Geometry: final body of the model. Coordinates: model frame, mm. A direction names the side the tool comes from. Give positions to 0.01 mm unless a question says otherwise; leave off trailing zeros. Loops run counter-clockwise (first coordinate to the right, second up) from the corner with the lowest first, then second, coordinate; pieces in that order, holes last.
from build123d import *

# Parameters (mm, degrees)
EXTRUDE_1_DEPTH = 4.5


with BuildPart() as part:
    # 草图1 → 凸台-拉伸1 (new body)
    with BuildSketch(Plane(origin=(0, 0, 0), x_dir=(1, 0, 0), z_dir=(0, 1, 0))):
        with BuildLine():
            Line((-6.23452468, 62.552230204), (0.89047532, 62.552230204))
            Line((0.89047532, 62.552230204), (0.89047532, 67.052230204))
            Line((0.89047532, 67.052230204), (8.01547532, 67.052230204))
            Line((8.01547532, 67.052230204), (8.01547532, 62.552230204))
            Line((8.01547532, 62.552230204), (15.14047532, 62.552230204))
            Line((15.14047532, 62.552230204), (15.14047532, 67.052230204))
            Line((15.14047532, 67.052230204), (22.26547532, 67.052230204))
            Line((22.26547532, 67.052230204), (22.26547532, 62.552230204))
            Line((22.26547532, 62.552230204), (29.39047532, 62.552230204))
            Line((29.39047532, 62.552230204), (29.39047532, 55.427230204))
            Line((29.39047532, 55.427230204), (33.89047532, 55.427230204))
            Line((33.89047532, 55.427230204), (33.89047532, 48.302230204))
            Line((33.89047532, 48.302230204), (29.39047532, 48.302230204))
            Line((29.39047532, 48.302230204), (29.39047532, 41.177230204))
            Line((29.39047532, 41.177230204), (33.89047532, 41.177230204))
            Line((33.89047532, 41.177230204), (33.89047532, 34.052230204))
            Line((33.89047532, 34.052230204), (29.39047532, 34.052230204))
            Line((29.39047532, 34.052230204), (29.39047532, 26.927230204))
            Line((29.39047532, 26.927230204), (33.89047532, 26.927230204))
            Line((33.89047532, 26.927230204), (33.89047532, 19.802230204))
            Line((33.89047532, 19.802230204), (29.39047532, 19.802230204))
            Line((29.39047532, 19.802230204), (29.39047532, 12.677230204))
            Line((29.39047532, 12.677230204), (33.89047532, 12.677230204))
            Line((33.89047532, 12.677230204), (33.89047532, 5.552230204))
            Line((33.89047532, 5.552230204), (29.39047532, 5.552230204))
            Line((29.39047532, 5.552230204), (29.39047532, -34.999800679))
            ThreePointArc((29.39047532, -34.999800679), (29.238234385, -35.765167544), (28.804688882, -36.414014242))
            Line((28.804688882, -36.414014242), (28.476261758, -36.742441366))
            ThreePointArc((28.476261758, -36.742441366), (28.042716255, -37.391288064), (27.89047532, -38.156654929))
            Line((27.89047532, -38.156654929), (27.89047532, -49.877331374))
            ThreePointArc((27.89047532, -49.877331374), (27.789489805, -50.877159896), (27.49061249, -51.83660114))
            Line((27.49061249, -51.83660114), (23.222752356, -61.857039562))
            ThreePointArc((23.222752356, -61.857039562), (21.379756021, -64.068881688), (18.622615186, -64.897769796))
            Line((18.622615186, -64.897769796), (-16.841664546, -64.897769796))
            ThreePointArc((-16.841664546, -64.897769796), (-19.598805381, -64.068881688), (-21.441801716, -61.857039562))
            Line((-21.441801716, -61.857039562), (-25.70966185, -51.83660114))
            ThreePointArc((-25.70966185, -51.83660114), (-26.008539165, -50.877159896), (-26.10952468, -49.877331374))
            Line((-26.10952468, -49.877331374), (-26.10952468, -38.156654929))
            ThreePointArc((-26.10952468, -38.156654929), (-26.261765615, -37.391288064), (-26.695311118, -36.742441366))
            Line((-26.695311118, -36.742441366), (-27.023738242, -36.414014242))
            ThreePointArc((-27.023738242, -36.414014242), (-27.457283745, -35.765167544), (-27.60952468, -34.999800679))
            Line((-27.60952468, -34.999800679), (-27.60952468, 5.552230204))
            Line((-27.60952468, 5.552230204), (-32.10952468, 5.552230204))
            Line((-32.10952468, 5.552230204), (-32.10952468, 12.677230204))
            Line((-32.10952468, 12.677230204), (-27.60952468, 12.677230204))
            Line((-27.60952468, 12.677230204), (-27.60952468, 19.802230204))
            Line((-27.60952468, 19.802230204), (-32.10952468, 19.802230204))
            Line((-32.10952468, 19.802230204), (-32.10952468, 26.927230204))
            Line((-32.10952468, 26.927230204), (-27.60952468, 26.927230204))
            Line((-27.60952468, 26.927230204), (-27.60952468, 34.052230204))
            Line((-27.60952468, 34.052230204), (-32.10952468, 34.052230204))
            Line((-32.10952468, 34.052230204), (-32.10952468, 41.177230204))
            Line((-32.10952468, 41.177230204), (-27.60952468, 41.177230204))
            Line((-27.60952468, 41.177230204), (-27.60952468, 48.302230204))
            Line((-27.60952468, 48.302230204), (-32.10952468, 48.302230204))
            Line((-32.10952468, 48.302230204), (-32.10952468, 55.427230204))
            Line((-32.10952468, 55.427230204), (-27.60952468, 55.427230204))
            Line((-27.60952468, 55.427230204), (-27.60952468, 67.052230204))
            Line((-27.60952468, 67.052230204), (-20.48452468, 67.052230204))
            Line((-20.48452468, 67.052230204), (-20.48452468, 62.552230204))
            Line((-20.48452468, 62.552230204), (-13.35952468, 62.552230204))
            Line((-13.35952468, 62.552230204), (-13.35952468, 67.052230204))
            Line((-13.35952468, 67.052230204), (-6.23452468, 67.052230204))
            Line((-6.23452468, 67.052230204), (-6.23452468, 62.552230204))
        make_face()
    extrude(amount=EXTRUDE_1_DEPTH)


solid = part.part
Item 1: Set-up query: faces 5 (the face through (29.39, 2, 14)), 6 (the face through (-30, 2, -12.677)), 7 (the face through (22.265, 2, -65)), 8 (the face through (32, 2, -12.677)), 9 (the face through (8.015, 2, -65)). Return all of +Z, -Z, +X, -X, +Y, -Y with unobstructed straight access to the full face (end or side cutting, diameter ignored); none if empty.
Values follow:
face 5: +Z, +X, +Y, -Y
face 6: -X, +Y, -Y
face 7: -Z, +X, +Y, -Y
face 8: +X, +Y, -Y
face 9: -Z, +Y, -Y
Item 2: Section query A-A on z = -30. Return loops of the section in (x, y).
Values follow:
outline: (-27.61, 0) - (29.39, 0) - (29.39, 4.5) - (-27.61, 4.5) - close
Item 3: Ray query, probe 1 along Z at (x, y) = (30.5, 1.3); probe 2 along X at (y, z) = (0.85, -3); probe 3 along Z at (x, y) = (8.5, 3.75). Return the intervals inside material, ascending.
Values follow:
probe 1: z = -55.43 to -48.3, -41.18 to -34.05, -26.93 to -19.8, -12.68 to -5.55
probe 2: x = -27.61 to 29.39
probe 3: z = -62.55 to 64.9
Item 4: Section query B-B on x = -15.5. Return loops of the section in (y, z), plus the area to 3 significant figures.
Values follow:
outline: (0, -62.55) - (4.5, -62.55) - (4.5, 64.9) - (0, 64.9) - close
area: 574 mm2
Item 5: Pin query (flat end, axial travel): pin 1 (2 mm diameter, centred on x = 31.5, y = 2, fed in from +Z); pin 2 (2 mm diameter, centred on y = 3, z = -30, fed in from -X); pin 3 (2 mm diameter, centred on y = 2, z = 51, fed in from -X). Return the tip coordinate at first contact, or that it passes through.
Values follow:
pin 1: stops at z = -5.55
pin 2: stops at x = -27.61
pin 3: stops at x = -26.11
Item 6: Draft query along Z for faces 1 (the face through (-27.61, 2, -45)), 2 (the face through (26, 2, -62.552)), 3 (the face through (-30, 2, -5.552)), 4 (the face through (0.89, 2, -65)). Return one class per face: +Z half, -Z half, draft (parallel to the pull), parting line (faces both ways), or undercut.
Values follow:
face 1: undercut
face 2: -Z half
face 3: +Z half
face 4: draft
